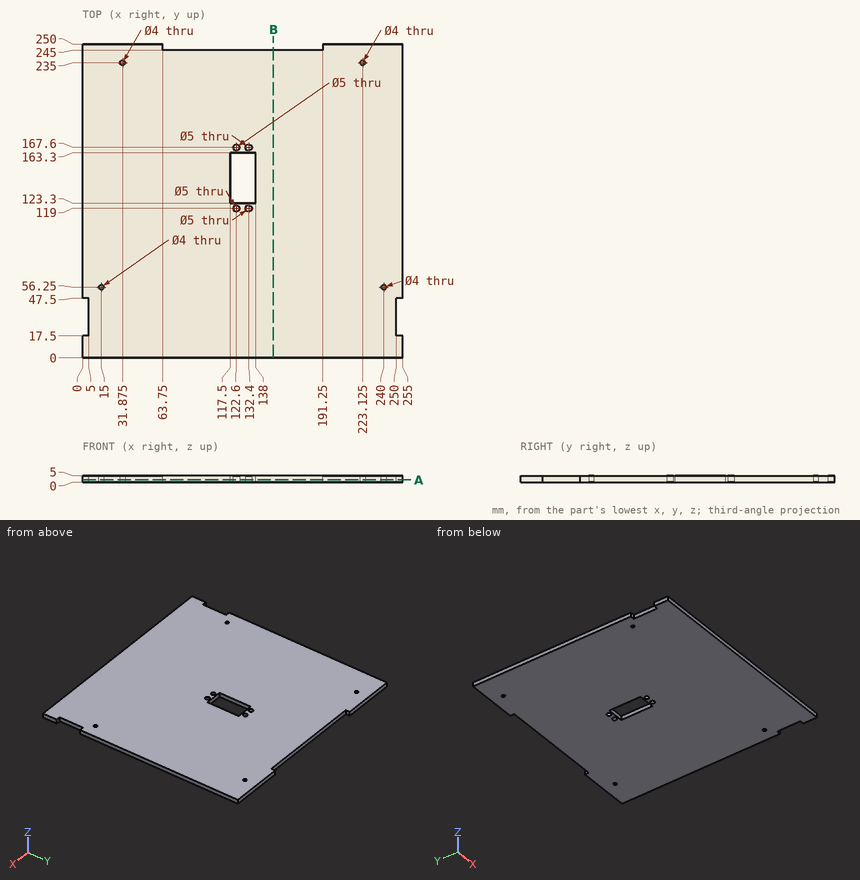
Geometry check sheet. Reference: drawing and pictorial views, mm from the part's lowest x, y, z. Give positions to 0.01 mm unless a question says otherwise; leave off trailing zeros. Loops run counter-clockwise (first coordinate to the right, second up) from the corner with the lowest first, then second, coordinate; pieces in that order, holes last. Notation, with made-up numbers: (14.5, 38.25) - (49.5, 38.25) arc R16 cw to (49.5, 55.25) - close; hole circle Ø11 at (44, -12). An arc over 180 degrees is marked (long way). One line per question, with ' | ' between items. Start each with the question number.
1. Cross-section at B-B, the plane x = 152. Enter the section's corners in (y, z).
2. Material ranges on line 1 along X through (y, z) = (235, 3.85) (3 decimals); line 2 along Y through (x, z) = (132.4, 3.35); line 3 along X through (y, z) = (167, 3.25), recorded low to high. Write a range as [from, to].
3. Gauge pin test, flat end, axial feed: pin 1 Ø4.5 at (x, y) = (122.6, 119) entering from -Z. Record the tip position at first contact, or that the pin passes through.
4. Cross-section at A-A, the plane z = 1.8. Give the number of separate pieces and of enclosed holes in the cut face, plus the area to 3 significant figures.
Check result:
1) outline: (0, 0) - (245, 0) - (245, 5) - (0, 5) - close
2) line 1: x = [0, 29.875], [33.875, 221.125], [225.125, 255] | line 2: y = [0, 116.5], [121.5, 123.3], [163.3, 165.1], [170.1, 245] | line 3: x = [0, 120.17], [125.03, 129.97], [134.83, 255]
3) pin 1: passes through
4) separate pieces: 1 | enclosed holes: 9 | area: 61,900 mm2
